Design review of the part built by this model. Coordinates are the model's own, in mm. A direction names the side the tool comes from. Give positions to 0.01 mm unless a question says otherwise; leave off trailing zeros. Loops run counter-clockwise (first coordinate to the right, second up) from the corner with the lowest first, then second, coordinate; pieces in that order, holes last. Notation, with made-up numbers: (72.5, 50.25) -> (77.5, 50.25) arc R38 cw to (77.5, 88.25) -> close; hole circle Ø2 at (3.25, 3). An arc over 180 degrees is marked (long way). Use CSV: the item, a comma, the result in double quotes. Start each with the question number.
Item 1: We need section C-C (z = 1). State the section outline as (x, y) points.
Item 2: We need section D-D (x = 0). State the section outline as (y, z) points.
Item 3: Wall thickness on line 1 along Z through (x, y) = (0, 6.5); line 2 along X through (y, z) = (7.4, 0); line 3 along Y through (x, z) = (15, -15.8): over which ranges is each line inside the solid? List them lowest first. Write a range as from..to.
Item 4: We need section A-A (x = 15). State the section outline as (y, z) points.
Item 5: The part is to be moulded in two halves that separate along Z. For faces 1 (the face through (2, 4, -12)), 2 (the face through (18, 4, -16)), 3 (the face through (0, 4, -18)), say which applies: +Z half, -Z half, draft (parallel to the pull), parting line (faces both ways), or undercut.
Item 6: Clearance check with flat-ended pins moving along their axes: pin 1 (1.5 mm diameter, centred on x = 10.5, y = 1.5, fed in from +Z); pin 2 (1.5 mm diameter, centred on y = 5.5, z = -11, fed in from -X); pin 3 (6 mm diameter, centred on y = 4.5, z = 5, fed in from -X); pin 4 (2.5 mm diameter, centred on x = 0, z = 0, fed in from +Y). State where each tip first meets the part, or that it passes through.
Item 7: For faces 4 (the face through (-16.5, 3.8, -16.5)), 5 (the face through (7.62, 6.96, 3.16)), 6 (the face through (-18, 4, -17)), 7 (the face through (-2.6, 4.06, -14.43)), 8 (the face through (11, 4, -15)), list the 3-axis set-ups (+Z, -Z, +X, -X, +Y, -Y) from which the entire face can be reached by the end or side of a thin tool; tool diameter is ignored.
Item 8: We need section B-B (y = 6). State the section outline as (x, z) points.
from build123d import *

# Parameters (mm, degrees)
SKETCH_1_R          = 8.75
SKETCH_1_R_2        = 8.25
EXTRUDE_2_DEPTH     = 10
SKETCH_2_R          = 8.25
SKETCH_2_R_2        = 2
EXTRUDE_3_DEPTH     = 4
EXTRUDE_4_DEPTH     = 8
SKETCH_5_W          = 3
SKETCH_5_H          = 8
EXTRUDE_5_DEPTH     = 3
SKETCH_6_W          = 3
SKETCH_6_H          = 8
EXTRUDE_6_DEPTH     = 3
SKETCH_7_R          = 1.5
CUT_EXTRUDE_1_DEPTH = 3
FILLET_1_R          = 5
FILLET_3_R          = 2
SKETCH_8_R          = 8.75
SKETCH_8_R_2        = 8.25
EXTRUDE_7_DEPTH     = 8
SKETCH_9_R          = 8.25
SKETCH_9_R_2        = 6
EXTRUDE_8_DEPTH     = 2
EXTRUDE_9_DEPTH     = 8
SKETCH_11_R         = 1.5
CUT_EXTRUDE_2_DEPTH = 8
CUT_EXTRUDE_3_DEPTH = 8
CUT_EXTRUDE_4_DEPTH = 8
SKETCH_14_R         = 8.75
SKETCH_14_R_2       = 8.25
EXTRUDE_10_DEPTH    = 8
EXTRUDE_11_DEPTH    = 8
SKETCH_16_R         = 1.5
CUT_EXTRUDE_5_DEPTH = 8
CUT_EXTRUDE_6_DEPTH = 10


with BuildPart() as part:
    # 草图1 → 凸台-拉伸2 (new body)
    with BuildSketch(Plane(origin=(0, 0, 0), x_dir=(1, 0, 0), z_dir=(0, 1, 0))):
        Circle(SKETCH_1_R)
        Circle(SKETCH_1_R_2, mode=Mode.SUBTRACT)
    extrude(amount=EXTRUDE_2_DEPTH)

    # 草图2 → 凸台-拉伸3 (add)
    with BuildSketch(Plane(origin=(0, 0, 0), x_dir=(1, 0, 0), z_dir=(0, 1, 0))):
        Circle(SKETCH_2_R)
        Circle(SKETCH_2_R_2, mode=Mode.SUBTRACT)
    extrude(amount=EXTRUDE_3_DEPTH)

    # 草图3 → 凸台-拉伸4 (add)
    with BuildSketch(Plane(origin=(0, 0, 0), x_dir=(1, 0, 0), z_dir=(0, 1, 0))):
        Polygon((-2, 8.518362519), (2, 8.518362519), (2, 15), (15, 15), (15, 18), (2, 18), (-2, 18), (-15, 18), (-15, 15), (-2, 15), align=None)
    extrude(amount=EXTRUDE_4_DEPTH)

    # 草图5 → 凸台-拉伸5 (add)
    with BuildSketch(Plane(origin=(15, 0, 0), x_dir=(0, 0, -1), z_dir=(1, 0, 0))):
        with Locations((16.5, 4)):
            Rectangle(SKETCH_5_W, SKETCH_5_H)
    extrude(amount=EXTRUDE_5_DEPTH)

    # 草图6 → 凸台-拉伸6 (add)
    with BuildSketch(Plane.ZY.offset(15)):
        with Locations((-16.5, 4)):
            Rectangle(SKETCH_6_W, SKETCH_6_H)
    extrude(amount=EXTRUDE_6_DEPTH)

    # 草图7 → 切除-拉伸1 (cut)
    with BuildSketch(Plane(origin=(0, 0, -18), x_dir=(-1, 0, 0), z_dir=(0, 0, -1))):
        with Locations((-15, 3.754021035)):
            Circle(SKETCH_7_R)
    cut_extrude_1 = extrude(amount=-CUT_EXTRUDE_1_DEPTH, mode=Mode.SUBTRACT)

    # 镜向1: 切除-拉伸1 across plane
    add(cut_extrude_1.mirror(Plane(origin=(0, 0, 0), x_dir=(0, 0, 1), z_dir=(1, 0, 0))), mode=Mode.SUBTRACT)

    # 圆角1
    fillet_1_edges = [part.edges().sort_by_distance(p)[0] for p in [
        (-2, 4, -8.518362519),
        (2, 4, -8.518362519),
    ]]
    fillet(fillet_1_edges, radius=FILLET_1_R)

    # 圆角3
    fillet_3_edges = [part.edges().sort_by_distance(p)[0] for p in [
        (-2, 4, -15),
        (2, 4, -15),
    ]]
    fillet(fillet_3_edges, radius=FILLET_3_R)


with BuildPart() as body_2:
    # 草图8 → 凸台-拉伸7 (new body)
    with BuildSketch(Plane(origin=(0, 0, 0), x_dir=(1, 0, 0), z_dir=(0, 1, 0))):
        with Locations((27.184954533, 0)):
            Circle(SKETCH_8_R)
        with Locations((27.184954533, 0)):
            Circle(SKETCH_8_R_2, mode=Mode.SUBTRACT)
    extrude(amount=EXTRUDE_7_DEPTH)

    # 草图9 → 凸台-拉伸8 (add)
    with BuildSketch(Plane.XZ):
        with Locations((27.184954533, 0)):
            Circle(SKETCH_9_R)
        with Locations((27.184954533, 0)):
            Circle(SKETCH_9_R_2, mode=Mode.SUBTRACT)
    extrude(amount=-EXTRUDE_8_DEPTH)

    # 草图10 → 凸台-拉伸9 (add)
    with BuildSketch(Plane(origin=(0, 0, 0), x_dir=(1, 0, 0), z_dir=(0, 1, 0))):
        Polygon((27.184954533, -18), (45.184954533, -18), (45.184954533, -14.663867829), (29.184954533, -14.663867829), (29.184954533, -8.518362519), (25.184954533, -8.518362519), (25.184954533, -14.663867829), (9.184954533, -14.663867829), (9.184954533, -18), align=None)
    extrude(amount=EXTRUDE_9_DEPTH)

    # 草图11 → 切除-拉伸2 (cut)
    with BuildSketch(Plane.XY.offset(18)):
        with Locations((12.184954533, 4)):
            Circle(SKETCH_11_R)
        with Locations((42.184954533, 4)):
            Circle(SKETCH_11_R)
    extrude(amount=-CUT_EXTRUDE_2_DEPTH, mode=Mode.SUBTRACT)

    # 草图12 → 切除-拉伸3 (cut)
    with BuildSketch(Plane.XY.offset(18)):
        with BuildLine():
            Line((10.684954533, 4), (10.684954533, 5))
            ThreePointArc((10.684954533, 5), (12.184954533, 6.5), (13.684954533, 5))
            Line((13.684954533, 5), (13.684954533, 4))
            Line((13.684954533, 4), (13.684954533, 3))
            ThreePointArc((13.684954533, 3), (12.184954533, 1.5), (10.684954533, 3))
            Line((10.684954533, 3), (10.684954533, 4))
        make_face()
    extrude(amount=-CUT_EXTRUDE_3_DEPTH, mode=Mode.SUBTRACT)

    # 草图13 → 切除-拉伸4 (cut)
    with BuildSketch(Plane.XY.offset(18)):
        with BuildLine():
            Line((40.684954533, 4), (40.684954533, 5))
            ThreePointArc((40.684954533, 5), (42.184954533, 6.5), (43.684954533, 5))
            Line((43.684954533, 5), (43.684954533, 4))
            Line((43.684954533, 4), (43.684954533, 3))
            ThreePointArc((43.684954533, 3), (42.184954533, 1.5), (40.684954533, 3))
            Line((40.684954533, 3), (40.684954533, 4))
        make_face()
    extrude(amount=-CUT_EXTRUDE_4_DEPTH, mode=Mode.SUBTRACT)


with BuildPart() as body_3:
    # 草图14 → 凸台-拉伸10 (new body)
    with BuildSketch(Plane(origin=(0, 0, 0), x_dir=(1, 0, 0), z_dir=(0, 1, 0))):
        with Locations((-35.091635024, 0)):
            Circle(SKETCH_14_R)
        with Locations((-35.091635024, 0)):
            Circle(SKETCH_14_R_2, mode=Mode.SUBTRACT)
    extrude(amount=EXTRUDE_10_DEPTH)

    # 草图15 → 凸台-拉伸11 (add)
    with BuildSketch(Plane(origin=(0, 0, 0), x_dir=(1, 0, 0), z_dir=(0, 1, 0))):
        Polygon((-37.091635024, -15), (-37.091635024, -8.518362519), (-33.091635024, -8.518362519), (-33.091635024, -15), (-17.091635024, -15), (-17.091635024, -18), (-53.091635024, -18), (-53.091635024, -15), align=None)
    extrude(amount=EXTRUDE_11_DEPTH)

    # 草图16 → 切除-拉伸5 (cut)
    with BuildSketch(Plane.XY.offset(18)):
        with Locations((-50.091635024, 4)):
            Circle(SKETCH_16_R)
        with Locations((-20.091635024, 4)):
            Circle(SKETCH_16_R)
    extrude(amount=-CUT_EXTRUDE_5_DEPTH, mode=Mode.SUBTRACT)


with BuildPart() as cut_extrude_6_tool:
    # 草图17 → 切除-拉伸6 (new body)
    with BuildSketch(Plane(origin=(0, 0, 0), x_dir=(1, 0, 0), z_dir=(0, 1, 0))):
        Polygon((-33.937696103, 15.405684546), (-2.722219819, -15.809791737), (14.647012306, -5.078130135), (14.647012306, 8.915639327), (41.967984005, 12.760711076), (60.531615551, -22.761160297), (-4.034255232, -33.891518563), (-68.183747723, -30.767123944), (-78.804576394, -10.443960936), (-56.287548242, 12.073067216), align=None)
    extrude(amount=CUT_EXTRUDE_6_DEPTH)


with BuildPart() as body_2_1:
    add(body_2.part)

    # 切除-拉伸6: cut by cut_extrude_6_tool
    add(cut_extrude_6_tool.part, mode=Mode.SUBTRACT)


with BuildPart() as body_3_1:
    add(body_3.part)

    # 切除-拉伸6: cut by cut_extrude_6_tool
    add(cut_extrude_6_tool.part, mode=Mode.SUBTRACT)


solid = part.part
Results found:
1,outline,"(-8.69, 0) -> (-1.73, 0) -> (-1.73, 4) -> (-8.19, 4) -> (-8.19, 10) -> (-8.69, 10) -> close; (1.73, 0) -> (8.69, 0) -> (8.69, 10) -> (8.19, 10) -> (8.19, 4) -> (1.73, 4) -> close"
2,outline,"(0, -18) -> (8, -18) -> (8, -8.75) -> (10, -8.75) -> (10, -8.25) -> (4, -8.25) -> (4, -2) -> (0, -2) -> close; (0, 2) -> (4, 2) -> (4, 8.25) -> (10, 8.25) -> (10, 8.75) -> (0, 8.75) -> close"
3,line 1,"-18..-8.25, 8.25..8.75"
3,line 2,"-8.75..-8.25, 8.25..8.75"
3,line 3,"0..2.25, 5.25..8"
4,outline,"(0, -18) -> (2.25, -18) -> (2.25, -15) -> (0, -15) -> close; (5.25, -18) -> (8, -18) -> (8, -15) -> (5.25, -15) -> close"
5,face 1,"undercut"
5,face 2,"draft"
5,face 3,"-Z half"
6,pin 1,"z = -15"
6,pin 2,"x = -2.26"
6,pin 3,"x = -8.52"
6,pin 4,"through"
7,face 4,"+Z, -Z"
7,face 5,"+Y"
7,face 6,"+Z, -Z, -X, +Y, -Y"
7,face 7,"-X, +Y, -Y"
7,face 8,"+X, +Y, -Y"
8,outline,"(-18, -18) -> (18, -18) -> (18, -15) -> (4, -15) arc R2 cw to (2, -13) -> (2, -11.83) arc R5 cw to (4.45, -7.53) arc R8.75 ccw (long way) to (-4.45, -7.53) arc R5 cw to (-2, -11.83) -> (-2, -13) arc R2 cw to (-4, -15) -> (-18, -15) -> close; hole circle Ø16.5 at (0, 0)"
